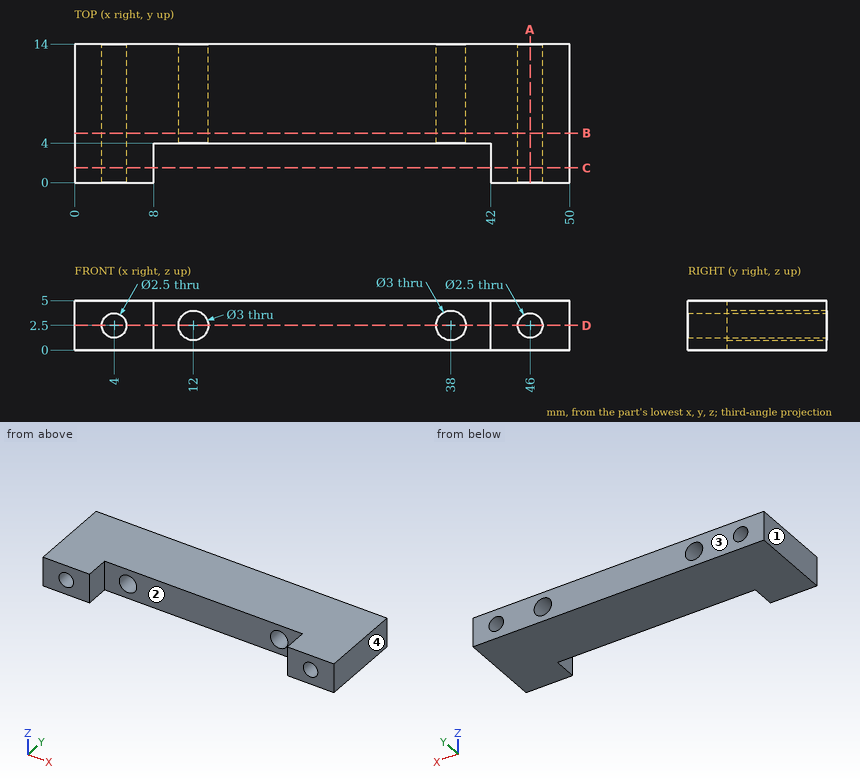
Could you check a few things on this drawing? It's one solid part, dimensions in mm from its lowest x, y, z. Give positions to 0.01 mm unless a question says otherwise; leave off trailing zeros. Order: outer loops, then holes, each group sorted by start corner. A loop starts at its lowest first (then second) coordinate and runs counter-clockwise, first axis right, second up.
1. Suppose I cut it at D-D (z = 2.5). Write out the boundary of the cut face in (x, y).
Answers below:
outline: (0, 0) - (2.75, 0) - (2.75, 14) - (0, 14) - close; (5.25, 0) - (8, 0) - (8, 4) - (10.5, 4) - (10.5, 14) - (5.25, 14) - close; (13.5, 4) - (36.5, 4) - (36.5, 14) - (13.5, 14) - close; (39.5, 4) - (42, 4) - (42, 0) - (44.75, 0) - (44.75, 14) - (39.5, 14) - close; (47.25, 0) - (50, 0) - (50, 14) - (47.25, 14) - close
2. Suppose I cut it at C-C (y = 1.5). Write out the boundary of the cut face in (x, z).
Answers below:
outline: (0, 0) - (8, 0) - (8, 5) - (0, 5) - close; (42, 0) - (50, 0) - (50, 5) - (42, 5) - close; hole circle Ø2.5 at (4, 2.5); hole circle Ø2.5 at (46, 2.5)
3. I need wall thicknesses on L1, parallel to Z at x = 4, y = 7.25; L2, parallel to X at y = 2.5, z = 1.75; L3, parallel to X at y = 11.75, z = 1.65. Which ranges of each line are inside material? Lowest first, please.
Answers below:
L1: z = 0 to 1.25, 3.75 to 5
L2: x = 0 to 3, 5 to 8, 42 to 45, 47 to 50
L3: x = 0 to 3.08, 4.92 to 10.76, 13.24 to 36.76, 39.24 to 45.08, 46.92 to 50
4. Suppose I cut it at B-B (y = 5). Write out the boundary of the cut face in (x, z), plus the area to 3 significant figures.
Answers below:
outline: (0, 0) - (50, 0) - (50, 5) - (0, 5) - close; hole circle Ø2.5 at (4, 2.5); hole circle Ø3 at (12, 2.5); hole circle Ø3 at (38, 2.5); hole circle Ø2.5 at (46, 2.5)
area: 226 mm2
5. For pin 1 (1.8 mm diameter, centred on x = 12, z = 2.5, fed in from +Y), with a flat end and sliding along its axis, tell me the tip position at first contact or that it passes through.
Answers below:
pin 1: passes through
6. Suppose I cut it at A-A (x = 46). Write out the boundary of the cut face in (y, z), plus the area to 3 significant figures.
Answers below:
outline: (0, 0) - (14, 0) - (14, 1.25) - (0, 1.25) - close; (0, 3.75) - (14, 3.75) - (14, 5) - (0, 5) - close
area: 35.0 mm2
7. Thinking about a two-plate mould opening in X: for the marked faces 1, 2, 3 and 4, which applies, +X half, -X half, draft (parallel to the pull), parting line (faces both ways), or undercut?
Answers below:
face 1: -X half
face 2: undercut
face 3: draft
face 4: +X half
